```python
from build123d import *

# Parameters (mm, degrees)
F0_W          = 63.5
F0_H          = 19.05
F1_DEPTH      = 5.08
F1_DEPTH_BACK = 5.08
F2_R          = 6.35
F3_DEPTH      = 25.4
F4_R          = 1.27


with BuildPart() as f1:
    # F0 (on Right) → F1 (new body, two sides)
    with BuildSketch(Plane.YZ) as f1_sk:
        Rectangle(F0_W, F0_H)
    extrude(amount=F1_DEPTH)
    extrude(f1_sk.sketch, amount=-F1_DEPTH_BACK)

    # F2 (on face) → F3 (cut)
    with BuildSketch(Plane.YZ.offset(5.08)):
        with Locations((22.606, 0)):
            Circle(F2_R)
        with Locations((-22.606, 0.390719)):
            Circle(F2_R)
    extrude(amount=-F3_DEPTH, mode=Mode.SUBTRACT)

    # F4
    f4_edges = [f1.edges().sort_by_distance(p)[0] for p in [
        (5.08, 0, 9.525),
        (0, -31.75, 9.525),
        (-5.08, 0, 9.525),
        (0, 31.75, 9.525),
        (5.08, 31.75, 0),
        (-5.08, 31.75, 0),
        (0, 31.75, -9.525),
        (0, -31.75, -9.525),
        (5.08, 0, -9.525),
        (-5.08, 0, -9.525),
        (5.08, -31.75, 0),
        (-5.08, -31.75, 0),
    ]]
    fillet(f4_edges, radius=F4_R)


solid = f1.part
```
Work out the finished part from the listing and answer in its coordinate system (mm). Round coordinates to 2 decimals unless told otherwise and drop trailing zeros. Order: outer loops, then holes, each group sorted by start corner. A loop starts at its lowest first (then second) coordinate and runs counter-clockwise, first axis right, second up.
Q1. Find the intervals of material crossed by line 1 along Y through (x, z) = (-1.5, 5.75); line 2 along Y through (x, z) = (0.25, -2); line 3 along Z through (x, y) = (3.5, 17.5) (3 decimals), in increasing order.
Solution:
line 1: y = -31.75 to -26.01, -19.2 to 19.91, 25.3 to 31.75
line 2: y = -31.75 to -28.49, -16.72 to 16.58, 28.63 to 31.75
line 3: z = -9.525 to -3.775, 3.775 to 9.525
Q2. The mould has two halves that part along Y. Classify faces 1 (the flat face through (0, 0, 9.525)), 2 (the cylindrical face through (0.05, 31.37, -9.16)), 3 (the cylindrical face through (0.07, 28.66, 1.91)), 4 (the cylindrical face through (0.07, -28.95, 0.67)): pulls with the +Y half, pulls with the -Y half, needs draft (parallel to the pull), parting line crosses it, or undercut.
Solution:
face 1: needs draft
face 2: pulls with the +Y half
face 3: undercut
face 4: undercut
Q3. A cutting plane is placed at C-C, the plane y = 26. Determine the outline of the cut face in (x, z) (3 decimals).
Solution:
outline: (-5.08, -8.255) arc R1.27 ccw to (-3.81, -9.525) - (3.81, -9.525) arc R1.27 ccw to (5.08, -8.255) - (5.08, -5.367) - (-5.08, -5.367) - close; (-5.08, 5.367) - (5.08, 5.367) - (5.08, 8.255) arc R1.27 ccw to (3.81, 9.525) - (-3.81, 9.525) arc R1.27 ccw to (-5.08, 8.255) - close
Q4. A cutting plane is placed at A-A, the plane y = -19. Determine the outline of the cut face in (x, z) (1 decimal).
Solution:
outline: (-5.1, -8.3) arc R1.3 ccw to (-3.8, -9.5) - (3.8, -9.5) arc R1.3 ccw to (5.1, -8.3) - (5.1, -4.8) - (-5.1, -4.8) - close; (-5.1, 5.6) - (5.1, 5.6) - (5.1, 8.3) arc R1.3 ccw to (3.8, 9.5) - (-3.8, 9.5) arc R1.3 ccw to (-5.1, 8.3) - close
Q5. A cutting plane is placed at B-B, the plane x = -0.5. Determine the outline of the cut face in (y, z) (3 decimals).
Solution:
outline: (-31.75, -8.255) arc R1.27 ccw to (-30.48, -9.525) - (30.48, -9.525) arc R1.27 ccw to (31.75, -8.255) - (31.75, 8.255) arc R1.27 ccw to (30.48, 9.525) - (-30.48, 9.525) arc R1.27 ccw to (-31.75, 8.255) - close; hole circle Ø12.7 at (-22.606, 0.391); hole circle Ø12.7 at (22.606, 0)
